```python
from build123d import *

# Parameters (mm, degrees)
F0_R     = 1.25
F1_DEPTH = 1.5


with BuildPart() as f1:
    # F0 (on Front) → F1 (new body)
    with BuildSketch(Plane.XZ):
        with BuildLine():
            Line((0.85, 38), (0, 39))
            Line((0, 39), (-0.85, 38))
            Line((-0.85, 38), (-2.5, -2))
            Line((-2.5, -2), (-7, -12))
            ThreePointArc((-7, -12), (-3.669946, -13.59481), (0, -14))
            ThreePointArc((0, -14), (3.669946, -13.59481), (7, -12))
            Line((7, -12), (2.5, -2))
            Line((2.5, -2), (0.85, 38))
        make_face()
        Circle(F0_R, mode=Mode.SUBTRACT)
    extrude(amount=F1_DEPTH)


solid = f1.part
```
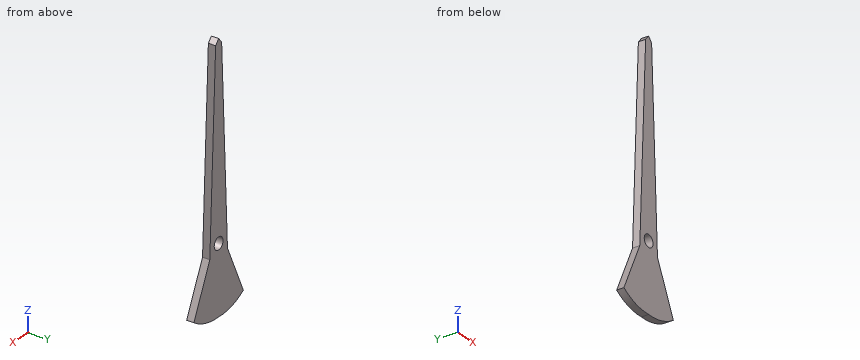
Input: part model. Units: mm. Frame: model coordinates. Coordinates: 2 decimals unless noted, no trailing zeros. Order: outer loops, then holes, each group sorted by start corner. A loop starts at its lowest first (then second) coordinate and runs counter-clockwise, first axis right, second up. Notation, with made-up numbers: (82, 24.5) - (126, 24.5) arc R16 cw to (126, 31.5) - close; hole circle Ø4 at (70.5, 35). An arc over 180 degrees is marked (long way). Put each result on its own line as item: value.
1. Line query: line 1 along Z through (x, y) = (0.25, -1.05); line 2 along X through (y, z) = (-1.3, 13.5); line 3 along Z through (x, y) = (-3.75, -1.2). Output: solid intervals per line, ascending.
Report:
line 1: z = -14.01 to -1.22, 1.22 to 38.71
line 2: x = -1.86 to 1.86
line 3: z = -13.57 to -4.78
2. Contact query for a flat-ended pin moving along its axis: pin 1 Ø2 at (x, z) = (-3.5, 28.5) entering from +Y. Output: stop coordinate, or through.
Report:
pin 1: passes through
3. Cut plane C-C on z = 30. Return the cut outline in (x, y), then the cut area to 3 significant figures.
Report:
outline: (-1.18, -1.5) - (1.18, -1.5) - (1.18, 0) - (-1.18, 0) - close
area: 3.54 mm2
4. Cut plane A-A on y = -0.5. Return the cut outline in (x, z), then the cut area to 3 significant figures.
Report:
outline: (-7, -12) arc R11.02 ccw to (0, -14) arc R11.02 ccw to (7, -12) - (2.5, -2) - (0.85, 38) - (0, 39) - (-0.85, 38) - (-2.5, -2) - close; hole circle Ø2.5 at (0, 0)
area: 245 mm2
5. Cut plane D-D on x = 4.25. Return the cut outline in (y, z), then the cut area to 3 significant figures.
Report:
outline: (-1.5, -13.41) - (0, -13.41) - (0, -5.89) - (-1.5, -5.89) - close
area: 11.3 mm2
6. Cut plane B-B on z = 0. Return the cut outline in (x, y), then the cut area to 3 significant figures.
Report:
outline: (-2.42, -1.5) - (-1.25, -1.5) - (-1.25, 0) - (-2.42, 0) - close; (1.25, -1.5) - (2.42, -1.5) - (2.42, 0) - (1.25, 0) - close
area: 3.50 mm2
